CAD build for the part. Positions are in the model's coordinates, mm. Face numbers are marked on the shaded views. Give positions to 0.01 mm unless a question says otherwise; leave off trailing zeros. Write each loop counter-clockwise with the first axis right and the second up, starting at its lowest first coordinate (ties: lowest second). Pieces come first, ordered by that corner, then holes. Notation, with made-up numbers: (-14, -5.75) - (31, -5.75) arc R17 ccw to (31, -0.75) - close; hole circle Ø7 at (69, 76). An arc over 180 degrees is marked (long way). Answer as a JSON object with one key per item and string values.
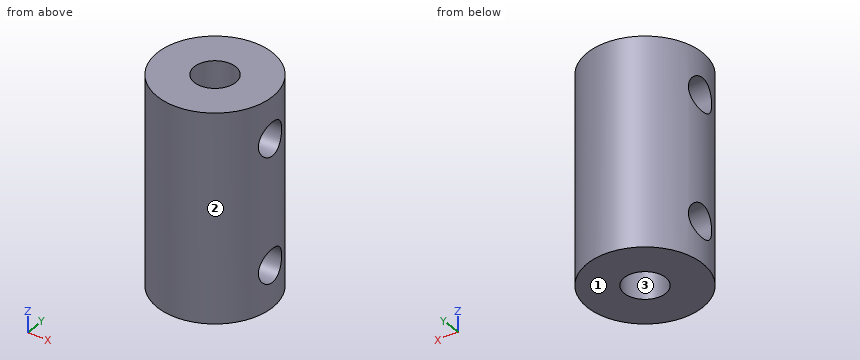
from build123d import *

# Parameters (mm, degrees)
SKETCH_1_R          = 6.95
SKETCH_1_R_2        = 2.5
EXTRUDE_1_DEPTH     = 25
SKETCH_2_R          = 2
CUT_EXTRUDE_1_DEPTH = 30.436584381


with BuildPart() as part:
    # 草图1 → 凸台-拉伸1 (new body)
    with BuildSketch(Plane.XY):
        Circle(SKETCH_1_R)
        Circle(SKETCH_1_R_2, mode=Mode.SUBTRACT)
    extrude(amount=EXTRUDE_1_DEPTH)

    # 草图2 → 切除-拉伸1 (cut, through all)
    with BuildSketch(Plane(origin=(6.95, 0, 0), x_dir=(0, 0, -1), z_dir=(1, 0, 0))):
        with Locations((-5, 0)):
            Circle(SKETCH_2_R)
        with Locations((-20, 0)):
            Circle(SKETCH_2_R)
    extrude(amount=-CUT_EXTRUDE_1_DEPTH, mode=Mode.SUBTRACT)


solid = part.part
Item 1: Cut at C-C (z = 19.5). Give the cut face in (x, y).
Entries:
{"outline": "(-6.67, -1.94) arc R6.95 ccw to (6.67, -1.94) - (1.58, -1.94) arc R2.5 cw to (-1.58, -1.94) - close; (-6.67, 1.94) - (-1.58, 1.94) arc R2.5 cw to (1.58, 1.94) - (6.67, 1.94) arc R6.95 ccw to start"}
Item 2: Cut at B-B (y = 0). Give the cut face in (x, z), and give its area (3 significant figures).
Entries:
{"outline": "(-6.95, 0) - (-2.5, 0) - (-2.5, 3) - (-6.95, 3) - close; (-6.95, 7) - (-2.5, 7) - (-2.5, 18) - (-6.95, 18) - close; (-6.95, 22) - (-2.5, 22) - (-2.5, 25) - (-6.95, 25) - close; (2.5, 0) - (6.95, 0) - (6.95, 3) - (2.5, 3) - close; (2.5, 7) - (6.95, 7) - (6.95, 18) - (2.5, 18) - close; (2.5, 22) - (6.95, 22) - (6.95, 25) - (2.5, 25) - close", "area": "151 mm2"}
Item 3: Mould opens along Y. For the marked faces 1, 2 and 3 say: +Y half, -Y half, draft (parallel to the pull), parting line (faces both ways), or undercut.
Entries:
{"face 1": "draft", "face 2": "parting line", "face 3": "undercut"}
Item 4: Probe line 1 (Z direction, x = 4.6, y = 0); line 2 (Y direction, x = 0, z = 18.75); line 3 (Y direction, x = -0.75, z = 17.5). List the from-to ranges inside material, lowest first. Write a range as from..to.
Entries:
{"line 1": "0..3, 7..18, 22..25", "line 2": "-6.95..-2.5, 2.5..6.95", "line 3": "-6.91..-2.38, 2.38..6.91"}
Item 5: Flat gauge pins, fed straight in: P1, Ø6, axis at y = -4.5, z = 16.5, coming from the +X side; P2, Ø5, axis at y = -3.5, z = 19.5, coming from the -X side; P3, Ø2.5, axis at y = 0, z = 20, coming from the +X side; P4, Ø3, axis at y = -2, z = 8, coming from the -X side. Where does each tip first touch, or does it go through?
Entries:
{"P1": "x = 6.79", "P2": "x = -6.84", "P3": "through", "P4": "x = -6.93"}
Item 6: Cut at A-A (x = 0). Give the cut face in (y, z).
Entries:
{"outline": "(-6.95, 0) - (-2.5, 0) - (-2.5, 25) - (-6.95, 25) - close; (2.5, 0) - (6.95, 0) - (6.95, 25) - (2.5, 25) - close"}
Item 7: Cut at D-D (x = 3.5). Give the cut face in (y, z), and give its area (3 significant figures).
Entries:
{"outline": "(-6, 0) - (6, 0) - (6, 25) - (-6, 25) - close; hole circle Ø4 at (0, 5); hole circle Ø4 at (0, 20)", "area": "275 mm2"}
